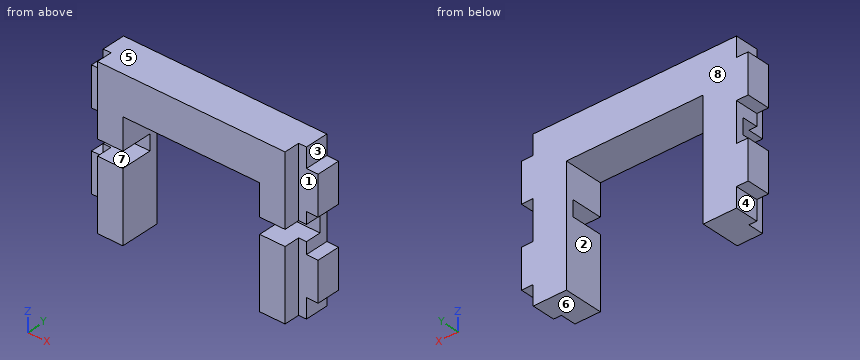
from build123d import *

# Parameters (mm, degrees)
BOSS_EXTRUDE1_DEPTH = 40
SKETCH2_W           = 35
SKETCH2_H           = 30
SKETCH2_W_2         = 3
SKETCH2_H_2         = 10
SKETCH2_H_3         = 5
CUT_EXTRUDE1_DEPTH  = 51.408332645
SKETCH3_W           = 58
SKETCH3_H           = 4
CUT_EXTRUDE2_DEPTH  = 8


with BuildPart() as part:
    # Sketch1 → Boss-Extrude1 (new body)
    with BuildSketch(Plane.XY):
        Polygon((24, -3), (29, -3), (29, 3), (-29, 3), (-29, -3), (-24, -3), (-24, -7), (24, -7), align=None)
    extrude(amount=BOSS_EXTRUDE1_DEPTH)

    # Sketch2 → Cut-Extrude1 (cut, through all)
    with BuildSketch(Plane(origin=(0, 3, 0), x_dir=(1, 0, 0), z_dir=(0, 1, 0))):
        with Locations((0, -15)):
            Rectangle(SKETCH2_W, SKETCH2_H)
        with Locations((27.5, -20)):
            Rectangle(SKETCH2_W_2, SKETCH2_H_2)
        with Locations((-27.5, -20)):
            Rectangle(SKETCH2_W_2, SKETCH2_H_2)
        with Locations((27.5, -37.5)):
            Rectangle(SKETCH2_W_2, SKETCH2_H_3)
        with Locations((-27.5, -37.5)):
            Rectangle(SKETCH2_W_2, SKETCH2_H_3)
        with Locations((-82.5, -20)):
            Rectangle(SKETCH2_W_2, SKETCH2_H_2)
        with Locations((27.5, 0)):
            Rectangle(SKETCH2_W_2, SKETCH2_H_2)
        with Locations((-27.5, 0)):
            Rectangle(SKETCH2_W_2, SKETCH2_H_2)
        with Locations((-82.5, 0)):
            Rectangle(SKETCH2_W_2, SKETCH2_H_2)
    extrude(amount=-CUT_EXTRUDE1_DEPTH, mode=Mode.SUBTRACT)

    # Sketch3 → Cut-Extrude2 (cut)
    with BuildSketch(Plane.XZ.offset(7)):
        with Locations((0, 20)):
            Rectangle(SKETCH3_W, SKETCH3_H)
    extrude(amount=-CUT_EXTRUDE2_DEPTH, mode=Mode.SUBTRACT)


solid = part.part
Geometry check sheet. Reference: the model listing, model coordinates, mm. Face numbers are marked on the shaded views. A direction names the side the tool comes from. Round coordinates to 2 decimals unless told otherwise and drop trailing zeros. Loops run counter-clockwise (first coordinate to the right, second up) from the corner with the lowest first, then second, coordinate; pieces in that order, holes last.
Item 1: Cross-section at D-D on z = 32.5. Record the boundary of the cut face in (x, y), then the cut area to 3 significant figures.
Item 2: Cross-section at B-B on z = 7.5. Record the boundary of the cut face in (x, y).
Item 3: Cross-section at C-C on x = 25. Record the boundary of the cut face in (y, z).
Item 4: Mould release check, pull along Z, two halves, no side actions. Record for the marked faces 5, 6, 7 and 8: pulls with the +Z half, pulls with the -Z half, needs draft (parallel to the pull), parting line crosses it, or undercut.
Item 5: Access from +Z, -Z, +X, -X, +Y, -Y to the whole of each face (thin tool, end or side, straight path). Record for the marked faces 1, 2, 3 and 4.
Item 6: Thickness scan on line 1 (Z direction, x = -23, y = 0); line 2 (X direction, y = 0.75, z = 10); line 3 (X direction, y = -2.25, z = 17). Record the ranges inside material, lowest first.
Item 7: Gauge pin test, flat ends, axial feed: pin 1 (3 mm diameter, centred on y = -1.5, z = 18, fed in from -X); pin 2 (1.5 mm diameter, centred on x = -17.5, y = -2, fed in from -Z); pin 3 (5.5 mm diameter, centred on x = -27, z = 12.5, fed in from -Y); pin 4 (0.9 mm diameter, centred on x = -27, y = -0.5, fed in from +Z). Record the tip position at first contact, or that the pin passes through.
Item 8: Cross-section at A-A on y = -1. Count the separate pieces of the cut face and the enclosed holes in it, then the cut area to 3 significant figures.
Answer sheet:
1. outline: (-29, -3) - (-24, -3) - (-24, -7) - (24, -7) - (24, -3) - (29, -3) - (29, 3) - (-29, 3) - close
1. area: 540 mm2
2. outline: (-29, -3) - (-24, -3) - (-24, -7) - (-17.5, -7) - (-17.5, 3) - (-29, 3) - close; (17.5, -7) - (24, -7) - (24, -3) - (29, -3) - (29, 3) - (17.5, 3) - close
3. outline: (-3, 0) - (3, 0) - (3, 40) - (-3, 40) - (-3, 22) - (1, 22) - (1, 18) - (-3, 18) - close
4. face 5: pulls with the +Z half
4. face 6: pulls with the -Z half
4. face 7: undercut
4. face 8: needs draft
5. face 1: +Z, -Z, +X, -Y
5. face 2: -Z, +Y, -Y
5. face 3: +Z, +X, +Y, -Y
5. face 4: -Z, -X, +Y, -Y
6. line 1: z = 0 to 18, 22 to 40
6. line 2: x = -29 to -17.5, 17.5 to 29
6. line 3: x = -26 to -17.5, 17.5 to 26
7. pin 1: stops at x = -26
7. pin 2: stops at z = 0
7. pin 3: stops at y = -3
7. pin 4: stops at z = 35
8. separate pieces: 3
8. enclosed holes: 0
8. area: 1,080 mm2
